from build123d import *

# Parameters (mm, degrees)
ESQUISSE1_W                                   = 30
ESQUISSE1_H                                   = 26
ESQUISSE1_R                                   = 11
BOSS_EXTRU_1_DEPTH                            = 10
TROU_POUR_TARAUDAGE_POUR_TROU_TARAUD_M2_D     = 1.6
TROU_POUR_TARAUDAGE_POUR_TROU_TARAUD_M2_DEPTH = 5
TROU_POUR_TARAUDAGE_POUR_TROU_TARAUD_M2_TIP   = 0.480688495
TROU_POUR_TARAUDAGE_POUR_TROU_TARAUD_2_D      = 1.6
TROU_POUR_TARAUDAGE_POUR_TROU_TARAUD_2_DEPTH  = 5
TROU_POUR_TARAUDAGE_POUR_TROU_TARAUD_2_TIP    = 0.480688495


with BuildPart() as part:
    # Esquisse1 → Boss.-Extru.1 (new body)
    with BuildSketch(Plane.XY):
        with Locations((15, 13)):
            Rectangle(ESQUISSE1_W, ESQUISSE1_H)
        with Locations((15, 13)):
            Circle(ESQUISSE1_R, mode=Mode.SUBTRACT)
    extrude(amount=BOSS_EXTRU_1_DEPTH)

    # Trou pour taraudage pour trou taraud_ M2
    with Locations(Plane(origin=(0, 26, 0), x_dir=(1, 0, 0), z_dir=(0, 1, 0))):
        with Locations((4, -5), (26, -5)):
            Hole(TROU_POUR_TARAUDAGE_POUR_TROU_TARAUD_M2_D / 2, depth=TROU_POUR_TARAUDAGE_POUR_TROU_TARAUD_M2_DEPTH)
            with Locations((0, 0, -(TROU_POUR_TARAUDAGE_POUR_TROU_TARAUD_M2_DEPTH + TROU_POUR_TARAUDAGE_POUR_TROU_TARAUD_M2_TIP / 2))):  # 118° drill point
                Cone(0, TROU_POUR_TARAUDAGE_POUR_TROU_TARAUD_M2_D / 2, TROU_POUR_TARAUDAGE_POUR_TROU_TARAUD_M2_TIP, mode=Mode.SUBTRACT)

    # Trou pour taraudage pour trou taraud 2
    with Locations(Plane(origin=(0, 0, 0), x_dir=(-1, 0, 0), z_dir=(0, -1, 0))):
        with Locations((-4, -5), (-26, -5)):
            Hole(TROU_POUR_TARAUDAGE_POUR_TROU_TARAUD_2_D / 2, depth=TROU_POUR_TARAUDAGE_POUR_TROU_TARAUD_2_DEPTH)
            with Locations((0, 0, -(TROU_POUR_TARAUDAGE_POUR_TROU_TARAUD_2_DEPTH + TROU_POUR_TARAUDAGE_POUR_TROU_TARAUD_2_TIP / 2))):  # 118° drill point
                Cone(0, TROU_POUR_TARAUDAGE_POUR_TROU_TARAUD_2_D / 2, TROU_POUR_TARAUDAGE_POUR_TROU_TARAUD_2_TIP, mode=Mode.SUBTRACT)


solid = part.part
Geometry check sheet. Reference: the model listing, model coordinates, mm. A direction names the side the tool comes from. Give positions to 0.01 mm unless a question says otherwise; leave off trailing zeros. Order: outer loops, then holes, each group sorted by start corner. A loop starts at its lowest first (then second) coordinate and runs counter-clockwise, first axis right, second up.
1) Material ranges on probe 1 along Y at (x, z) = (15, 5.5); probe 2 along Z at (x, y) = (26, 22.35); probe 3 along X at (y, z) = (24.35, 5), recorded low to high.
Results are:
probe 1: y = 0 to 2, 24 to 26
probe 2: z = 0 to 4.2, 5.8 to 10
probe 3: x = 0 to 3.2, 4.8 to 25.2, 26.8 to 30
2) Cross-section at C-C (z = 2). Record the boundary of the cut face in (x, y), then the cut area to 3 significant figures.
Results are:
outline: (0, 0) - (30, 0) - (30, 26) - (0, 26) - close; hole circle Ø22 at (15, 13)
area: 400 mm2
3) Gauge pin test, flat ends, axial feed: pin 1 (2.5 mm diameter, centred on x = 4, z = 5, fed in from -Y); pin 2 (12 mm diameter, centred on x = 19, y = 14, fed in from -Z). Record the tip position at first contact, or that the pin passes through.
Results are:
pin 1: stops at y = 0
pin 2: passes through
4) Tool access check on faces 1 (the cylindrical face through (25.261, 23.465, 5.306)), 2 (the cylindrical face through (12.62, 2.26, 4.93)), 3 (the cylindrical face through (26.739, 2.535, 5.306)). Record the directions out of +Z, -Z, +X, -X, +Y, -Y that give a thin tool (end or side, any length) a straight path to the whole face; none if there is none.
Results are:
face 1: +Y
face 2: +Z, -Z
face 3: -Y
5) Cross-section at A-A (y = 13). Record the boundary of the cut face in (x, z).
Results are:
outline: (0, 0) - (4, 0) - (4, 10) - (0, 10) - close; (26, 0) - (30, 0) - (30, 10) - (26, 10) - close
6) Draft check along Z on faces 4 (the flat face through (0, 13, 5)), 5 (the conical face through (26.11, 5.4, 5.08)), 6 (the flat face through (8, 22, 10)). Enter one of: released by +Z, released by -Z, zero draft, split by the parting line, or undercut.
Results are:
face 4: zero draft
face 5: undercut
face 6: released by +Z
7) Cross-section at B-B (x = 15). Record the boundary of the cut face in (y, z), then the cut area to 3 significant figures.
Results are:
outline: (0, 0) - (2, 0) - (2, 10) - (0, 10) - close; (24, 0) - (26, 0) - (26, 10) - (24, 10) - close
area: 40.0 mm2
